```python
from build123d import *

# Parameters (mm, degrees)
F0_W     = 152.4
F0_H     = 76.2
F1_DEPTH = 38.1
F2_T     = -2.54
F3_W     = 30.8243110776
F3_H     = 7.8012128361
F3_W_2   = 6.2790252268
F3_H_2   = 30.0632109866
F3_W_3   = 30.8243031614
F3_H_3   = 28.7312981673
F3_W_4   = 8.3720344119
F3_H_4   = 29.8729380593
F3_W_5   = 31.2048504129
F3_W_6   = 6.0887485743
F3_H_5   = 29.6826614067
F3_W_7   = 30.443765223
F4_DEPTH = 38.1


with BuildPart() as f1:
    # F0 (on Top) → F1 (new body)
    with BuildSketch(Plane.XY):
        Rectangle(F0_W, F0_H)
    extrude(amount=F1_DEPTH)

    # F2
    f2_openings = [f1.faces().sort_by_distance(p)[0] for p in [
        (0, 0, 0),
    ]]
    offset(amount=F2_T, openings=f2_openings)

    # F3 (on Top) → F4 (join)
    with BuildSketch(Plane.XY):
        with Locations((-56.5112270415, -0.1902736258)):
            Rectangle(F3_W, F3_H)
        with Locations((-37.9595588893, -0.1902736258)):
            Rectangle(F3_W_2, F3_H)
        with Locations((-37.9595588893, -19.1224855371)):
            Rectangle(F3_W_2, F3_H_2)
        with Locations((-19.4078946952, -0.1902736258)):
            Rectangle(F3_W_3, F3_H)
        with Locations((-37.9595588893, 18.0759818759)):
            Rectangle(F3_W_2, F3_H_3)
        with Locations((0.1902740914, -0.1902736258)):
            Rectangle(F3_W_4, F3_H)
        with Locations((0.1902740914, -19.0273490734)):
            Rectangle(F3_W_4, F3_H_4)
        with Locations((19.9787165038, -0.1902736258)):
            Rectangle(F3_W_5, F3_H)
        with Locations((0.1902740914, 18.0759818759)):
            Rectangle(F3_W_4, F3_H_3)
        with Locations((38.6255159974, -0.1902736258)):
            Rectangle(F3_W_6, F3_H)
        with Locations((38.6255159974, -18.9322107472)):
            Rectangle(F3_W_6, F3_H_5)
        with Locations((56.8917728961, -0.1902736258)):
            Rectangle(F3_W_7, F3_H)
        with Locations((38.6255159974, 18.0759818759)):
            Rectangle(F3_W_6, F3_H_3)
    extrude(amount=F4_DEPTH)


solid = f1.part
```
Check sheet for the modelled part. Datum: model origin and axes. Units: mm. A direction names the side the tool comes from. Give positions to 0.01 mm unless a question says otherwise; leave off trailing zeros. Loops run counter-clockwise (first coordinate to the right, second up) from the corner with the lowest first, then second, coordinate; pieces in that order, holes last. Notation, with made-up numbers: M 6.25,69.5 L 21.25,69.5 A23 ccw 21.25,97.5 Z; hole C -34.75,57 d6. An arc over 180 degrees is marked long. Answer as CSV lines item,"result".
Item 1: Sectioned sample at D-D, the plane x = -1. Enter the section's corners in (y, z), then the cut area to 3 significant figures.
Reply:
outline,"M -38.1,0 L -35.56,0 L -35.56,35.56 L -33.96,35.56 L -33.96,0 L 32.44,0 L 32.44,35.56 L 35.56,35.56 L 35.56,0 L 38.1,0 L 38.1,38.1 L -38.1,38.1 Z"
area,"2,740 mm^2"
Item 2: Set-up check for faces 4 (the face through (73.66, 0, 18)), 5 (the face through (-1, 38.1, 19)): record each of +Z, -Z, +X, -X, +Y, -Y from which the full face is reachable in a straight line by a thin tool's end or side.
Reply:
face 4,"-Z"
face 5,"+Z, -Z, +X, -X, +Y"
Item 3: Sectioned sample at B-B, the plane z = 24.5. State how many separate pieces and enclosed holes the cut face has, then the cut area to 3 significant figures.
Reply:
separate pieces,"2"
enclosed holes,"1"
area,"3,470 mm^2"
Item 4: Scan lines: L1, parallel to Y at x = 22, z = 31; L2, parallel to X at y = -6.5, z = 23; L3, parallel to X at y = 0.5, z = 7. Record each from-to range of solid material in increasing order.
Reply:
L1,"-38.1 to -35.56, -4.09 to 3.71, 35.56 to 38.1"
L2,"-76.2 to -73.66, -41.1 to -34.82, -4 to 4.38, 35.58 to 41.67, 73.66 to 76.2"
L3,"-76.2 to -73.66, -71.92 to 72.11, 73.66 to 76.2"
Item 5: Sectioned sample at C-C, the plane x = -37.5. Enter the section's corners in (y, z), then the cut area to 3 significant figures.
Reply:
outline,"M -38.1,0 L -35.56,0 L -35.56,35.56 L -34.15,35.56 L -34.15,0 L 32.44,0 L 32.44,35.56 L 35.56,35.56 L 35.56,0 L 38.1,0 L 38.1,38.1 L -38.1,38.1 Z"
area,"2,740 mm^2"
Item 6: Sectioned sample at A-A, the plane y = 12.5. Enter the section's corners in (x, z), then the cut area to 3 significant figures.
Reply:
outline,"M -76.2,0 L -73.66,0 L -73.66,35.56 L -41.1,35.56 L -41.1,0 L -34.82,0 L -34.82,35.56 L -4,35.56 L -4,0 L 4.38,0 L 4.38,35.56 L 35.58,35.56 L 35.58,0 L 41.67,0 L 41.67,35.56 L 73.66,35.56 L 73.66,0 L 76.2,0 L 76.2,38.1 L -76.2,38.1 Z"
area,"1,310 mm^2"
Item 7: Draft check along X on faces 1 (the face through (76.2, -1, 19)), 2 (the face through (-1, 1, 38.1)), 3 (the face through (-1, -35.56, 18)). Enter one of: pulls with the +X half, pulls with the -X half, needs draft (parallel to the pull), parting line crosses it, or undercut.
Reply:
face 1,"pulls with the +X half"
face 2,"needs draft"
face 3,"undercut"
